Read the model definition and answer for the solid it produces. Units are mm, in the model's axes. Face numbers are marked on the shaded views. A direction names the side the tool comes from. Round coordinates to 2 decimals unless told otherwise and drop trailing zeros. Write each loop counter-clockwise with the first axis right and the second up, starting at its lowest first coordinate (ties: lowest second). Pieces come first, ordered by that corner, then holes. Notation, with made-up numbers: (20, 83) -> (53, 83) arc R21 ccw to (53, 98) -> close; hole circle Ø2 at (23, 44). An arc over 180 degrees is marked (long way). Return JSON: item names as keys, results as strings.
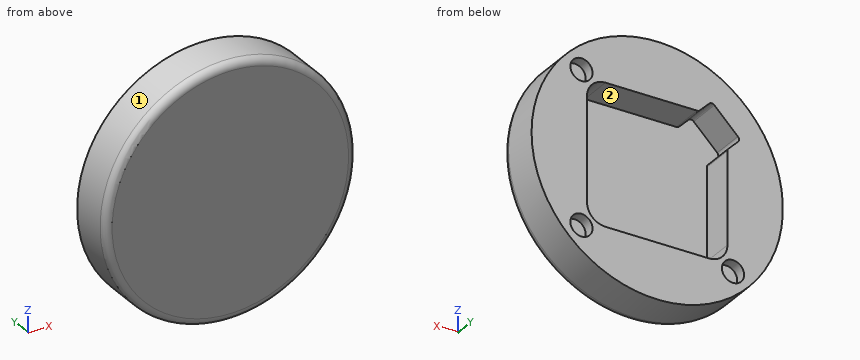
from build123d import *

# Parameters (mm, degrees)
SKETCH1_R           = 34
BOSS_EXTRUDE1_DEPTH = 3
SKETCH2_R           = 34
SKETCH2_W           = 38
SKETCH2_H           = 38
BOSS_EXTRUDE2_DEPTH = 9
FILLET1_R           = 5
SKETCH3_R           = 3
CUT_EXTRUDE1_DEPTH  = 3
CUT_EXTRUDE2_DEPTH  = 9
FILLET2_R           = 1
FILLET3_R           = 2


with BuildPart() as part:
    # Sketch1 → Boss-Extrude1 (new body)
    with BuildSketch(Plane(origin=(0, 0, 0), x_dir=(1, 0, 0), z_dir=(0, 1, 0))):
        Circle(SKETCH1_R)
    extrude(amount=BOSS_EXTRUDE1_DEPTH)

    # Sketch2 → Boss-Extrude2 (add)
    with BuildSketch(Plane(origin=(0, 3, 0), x_dir=(1, 0, 0), z_dir=(0, 1, 0))):
        Circle(SKETCH2_R)
        Rectangle(SKETCH2_W, SKETCH2_H, mode=Mode.SUBTRACT)
    extrude(amount=BOSS_EXTRUDE2_DEPTH)

    # Fillet1
    fillet1_edges = [part.edges().sort_by_distance(p)[0] for p in [
        (19, 7.5, -19),
        (-19, 7.5, -19),
        (-19, 7.5, 19),
        (19, 7.5, 19),
    ]]
    fillet(fillet1_edges, radius=FILLET1_R)

    # Sketch3 → Cut-Extrude1 (cut)
    with BuildSketch(Plane(origin=(0, 12, 0), x_dir=(1, 0, 0), z_dir=(0, 1, 0))):
        with Locations((-20.5, 20.512191497)):
            Circle(SKETCH3_R)
        with Locations((20.512191497, 20.5)):
            Circle(SKETCH3_R)
        with Locations((20.5, -20.512191497)):
            Circle(SKETCH3_R)
    extrude(amount=-CUT_EXTRUDE1_DEPTH, mode=Mode.SUBTRACT)

    # Sketch4 → Cut-Extrude2 (cut)
    with BuildSketch(Plane(origin=(0, 12, 0), x_dir=(1, 0, 0), z_dir=(0, 1, 0))):
        Polygon((-19, -11.221825407), (-22.535533906, -14.757359313), (-17.139357786, -20.153535433), (-14.757359313, -22.535533906), (-11.221825407, -19), align=None)
    extrude(amount=-CUT_EXTRUDE2_DEPTH, mode=Mode.SUBTRACT)

    # Fillet2
    fillet2_edges = [part.edges().sort_by_distance(p)[0] for p in [
        (-19, 7.5, 11.221825407),
        (-11.221825407, 7.5, 19),
        (-14.757359313, 7.5, 22.535533906),
        (-22.535533906, 7.5, 14.757359313),
    ]]
    fillet(fillet2_edges, radius=FILLET2_R)

    # Fillet3
    fillet3_edges = [part.edges().sort_by_distance(p)[0] for p in [
        (-34, 0, 0),
    ]]
    fillet(fillet3_edges, radius=FILLET3_R)


solid = part.part
Item 1: Section C-C (z = 0) is taken. Give the vertices of the cut face in (x, y).
Worked answers:
{"outline": "(-34, 2) arc R2 ccw to (-32, 0) -> (32, 0) arc R2 ccw to (34, 2) -> (34, 12) -> (19, 12) -> (19, 3) -> (-19, 3) -> (-19, 12) -> (-34, 12) -> close"}
Item 2: Straight lines are drawn through the part: L1, parallel to X at y = 3.75, z = -11.5; L2, parallel to X at y = 9.5, z = 18.5; L3, parallel to Z at x = 20.5, y = 10.7. For each, find the intervals that lie inside material, in ascending order. Write a range as [from, to].
Worked answers:
{"L1": "x = [-32, -19], [19, 32]", "L2": "x = [-28.53, -18.79], [16.18, 18.27], [22.73, 28.53]", "L3": "z = [-27.12, -23.5], [-17.5, 17.51], [23.51, 27.12]"}
Item 3: A tool of negligible diameter and unlimited length cuts with its end or side. For the marked faces 1 and 2, from which of +Z, -Z, +X, -X, +Y, -Y can it reach the whole face along a straight path? Write none if from no direction.
Worked answers:
{"face 1": "+Y, -Y", "face 2": "+Y"}
Item 4: Flat-ended cylindrical pins translate along their axes: pin 1 (1.5 mm diameter, centred on y = 9.5, z = 11.5, fed in from +X); pin 2 (8 mm diameter, centred on x = 20.51, z = -20.5, fed in from +Y); pin 3 (5 mm diameter, centred on x = -25.5, y = 5.5, fed in from -Z); pin 4 (7 mm diameter, centred on x = 1, y = 5.5, fed in from -Z). Find the tip coordinate at first contact, or state that the pin passes through.
Worked answers:
{"pin 1": "stops at x = 32.26", "pin 2": "stops at y = 12", "pin 3": "stops at z = -25.04", "pin 4": "stops at z = -34"}
Item 5: Section A-A (y = 5.5) is taken. Give the vertices of the cut face in (x, z), then the cut area to 3 significant figures.
Worked answers:
{"outline": "circle Ø68 at (0, 0); hole (-21.83, 14.05) -> (-19.29, 11.51) arc R1 cw to (-19, 10.81) -> (-19, -14) arc R5 ccw to (-14, -19) -> (14, -19) arc R5 ccw to (19, -14) -> (19, 14) arc R5 ccw to (14, 19) -> (-10.81, 19) arc R1 cw to (-11.51, 19.29) -> (-14.05, 21.83) arc R1 ccw to (-15.46, 21.83) -> (-21.83, 15.46) arc R1 ccw to start", "area": "2,180 mm2"}
Item 6: Section B-B (x = 0) is taken. Give the vertices of the cut face in (y, z), then the cut area to 3 significant figures.
Worked answers:
{"outline": "(0, -32) arc R2 ccw to (2, -34) -> (12, -34) -> (12, -19) -> (3, -19) -> (3, 19) -> (12, 19) -> (12, 34) -> (2, 34) arc R2 ccw to (0, 32) -> close", "area": "472 mm2"}
